Verification items for the finished model (mm, model axes). A direction names the side the tool comes from. Round coordinates to 2 decimals unless told otherwise and drop trailing zeros. Order: outer loops, then holes, each group sorted by start corner. A loop starts at its lowest first (then second) coordinate and runs counter-clockwise, first axis right, second up. Notation, with made-up numbers: M 66,80 L 85,80 A13 ccw 85,93 Z; hole C 32.5,62.25 d4. An arc over 180 degrees is marked long. Use CSV: the item, a comma, the result in double quotes. Start each with the question number.
Q1. Sectioned sample at B-B (x = -599.5). Enter the section's corners in (y, z), and give its area (3 significant figures).
Q2. Set-up check for faces 1 (the face through (-597, -850, -512)), 2 (the face through (-596.6, -863.6, -500.4)), 3 (the face through (-535.18, -830.563, -500.297)): record each of +Z, -Z, +X, -X, +Y, -Y from which the full face is reachable in a straight line by a thin tool's end or side.
Q3. Mould release check, pull along Y, two halves, no side actions. Record for faces 4 (the face through (-541.19, -845.72, -512.12)), 5 (the face through (-671.89, -837.675, -500.375)), 6 (the face through (-596.649, -863.496, -518.717)): +Y half, -Y half, draft (parallel to the pull), parting line (faces both ways), or undercut.
Q4. Scan lines: line 1 (Y direction, x = -589, z = -511.75); line 2 (Z direction, x = -603, y = -854.5); line 3 (Y direction, x = -555, z = -502.75). Record each from-to range of solid material in increasing order.
Q5. Sectioned sample at A-A (y = -831.5). Enter the section's corners in (x, z).
Q6. Sectioned sample at C-C (z = -511.75). Enter the section's corners in (x, y).
```python
from build123d import *

# Parameters (mm, degrees)
SKETCH014_W     = 151.632408
SKETCH014_H     = 21.2714
PAD009_DEPTH    = 40
SKETCH015_W     = 121.632408
SKETCH015_H     = 24
POCKET005_DEPTH = 21.2724
FILLET006_R     = 15
FILLET007_R     = 5


with BuildPart() as part:
    # Sketch014 (on Face1 of CopyPocket004) → Pad009 (new body)
    with BuildSketch(Plane.XZ.offset(825)):
        with Locations((-597.5, -509.507206)):
            Rectangle(SKETCH014_W, SKETCH014_H)
    extrude(amount=PAD009_DEPTH)

    # Sketch015 (on Face4 of Pad009) → Pocket005 (cut, through all)
    with BuildSketch(Plane(origin=(0, 0, -498.871506), x_dir=(-1, 0, 0), z_dir=(0, 0, 1))):
        with Locations((597.5, 838)):
            Rectangle(SKETCH015_W, SKETCH015_H)
    extrude(amount=-POCKET005_DEPTH, mode=Mode.SUBTRACT)

    # Fillet006
    fillet006_edges = [part.edges().sort_by_distance(p)[0] for p in [
        (-658.316204, -850, -509.507206),
        (-536.683796, -850, -509.507206),
        (-673.316204, -865, -509.507206),
        (-521.683796, -865, -509.507206),
    ]]
    fillet(fillet006_edges, radius=FILLET006_R)

    # Fillet007
    fillet007_edges = [part.edges().sort_by_distance(p)[0] for p in [
        (-597.5, -850, -498.871506),
        (-673.316204, -837.5, -498.871506),
        (-597.5, -865, -520.142906),
        (-673.316204, -837.5, -520.142906),
    ]]
    fillet(fillet007_edges, radius=FILLET007_R)


solid = part.part
```
Verdict:
1,outline,"M -865,-515.14 A5 ccw -860,-520.14 L -850,-520.14 L -850,-503.87 A5 ccw -855,-498.87 L -860,-498.87 A5 ccw -865,-503.87 Z; M -826,-520.14 L -825,-520.14 L -825,-498.87 L -826,-498.87 Z"
1,area,"324 mm²"
2,face 1,"+Z, -Z"
2,face 2,"+Z, +X, -X, -Y"
2,face 3,"+Z"
3,face 4,"undercut"
3,face 5,"draft"
3,face 6,"-Y half"
4,line 1,"y = -865 to -850, -826 to -825"
4,line 2,"z = -520.14 to -498.9"
4,line 3,"y = -864.87 to -850.13, -826 to -825"
5,outline,"M -673.32,-515.14 A5 ccw -668.32,-520.14 L -658.32,-520.14 L -658.32,-503.87 A5 ccw -663.32,-498.87 L -668.32,-498.87 A5 ccw -673.32,-503.87 Z; M -536.68,-520.14 L -526.68,-520.14 A5 ccw -521.68,-515.14 L -521.68,-503.87 A5 ccw -526.68,-498.87 L -531.68,-498.87 A5 ccw -536.68,-503.87 Z"
6,outline,"M -673.32,-850 A15 ccw -658.32,-865 L -536.68,-865 A15 ccw -521.68,-850 L -521.68,-825 L -673.32,-825 Z; hole M -658.32,-835 A15 ccw -643.32,-850 L -551.68,-850 A15 ccw -536.68,-835 L -536.68,-826 L -658.32,-826 Z"
